Verification items for this drawing (mm, ordinates from the low corner). Coordinates: 2 decimals unless noted, no trailing zeros. Write each loop counter-clockwise with the first axis right and the second up, starting at its lowest first coordinate (ties: lowest second). Pieces come first, ordered by that corner, then holes. Notation, with made-up numbers: (-40, 67) -> (0, 67) arc R5 ccw to (0, 74) -> close; hole circle Ø10 at (76.25, 89). An arc over 180 degrees is marked (long way). Put each result on its own line as item: value. Start each with the question number.
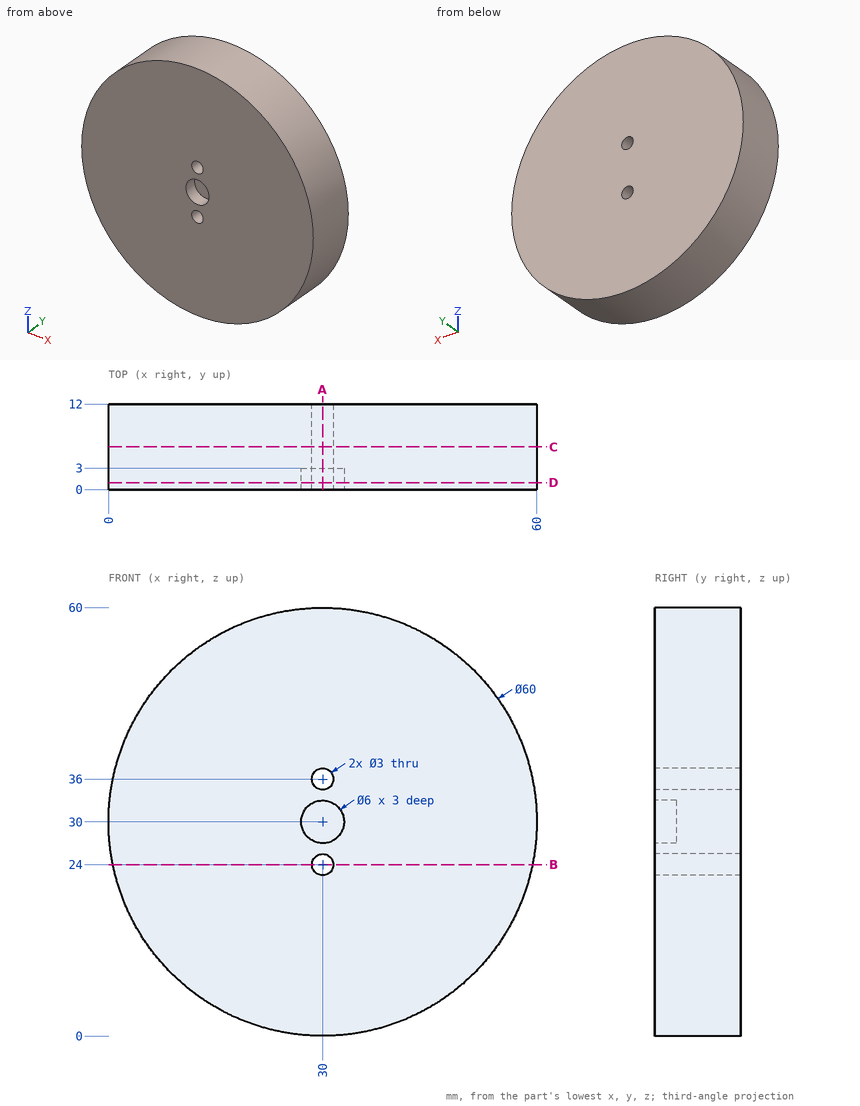
Item 1: Section check C-C, the plane y = 6. Enter the section's corners in (x, z), and give its area (3 significant figures).
Item 2: Section check D-D, the plane y = 1. Enter the section's corners in (x, z).
Item 3: Section check B-B, the plane z = 24. Enter the section's corners in (x, y), and give its area (3 significant figures).
Item 4: Go/stop test with flat-tipped pins: P1, Ø2, axis at y = 6, z = 47.5, coming from the +X side; P2, Ø1, axis at x = 51.5, y = 6.5, coming from the +Z side; P3, Ø1, axis at y = 4, z = 39.5, coming from the -X side; P4, Ø1.8, axis at x = 30, z = 24, coming from the +Y side. Record where each tip stops, or that it passes through.
Item 5: Scan lines: line 1 along Z through (x, y) = (30, 3.75); line 2 along Z through (x, y) = (30, 1); line 3 along Z through (x, y) = (38, 5.5). Record each from-to range of solid material in increasing order. Write a range as [from, to].
Item 6: Section check A-A, the plane x = 30. Enter the section's corners in (y, z).
From the geometry:
1. outline: circle Ø60 at (30, 30); hole circle Ø3 at (30, 24); hole circle Ø3 at (30, 36)
1. area: 2,810 mm²
2. outline: circle Ø60 at (30, 30); hole circle Ø6 at (30, 30); hole circle Ø3 at (30, 24); hole circle Ø3 at (30, 36)
3. outline: (0.61, 0) -> (28.5, 0) -> (28.5, 12) -> (0.61, 12) -> close; (31.5, 0) -> (59.39, 0) -> (59.39, 12) -> (31.5, 12) -> close
3. area: 669 mm²
4. P1: x = 55.05
4. P2: z = 51.42
4. P3: x = 1.38
4. P4: through
5. line 1: [0, 22.5], [25.5, 34.5], [37.5, 60]
5. line 2: [0, 22.5], [25.5, 27], [33, 34.5], [37.5, 60]
5. line 3: [1.09, 58.91]
6. outline: (0, 0) -> (12, 0) -> (12, 22.5) -> (0, 22.5) -> close; (0, 25.5) -> (12, 25.5) -> (12, 34.5) -> (0, 34.5) -> (0, 33) -> (3, 33) -> (3, 27) -> (0, 27) -> close; (0, 37.5) -> (12, 37.5) -> (12, 60) -> (0, 60) -> close
